Read the model definition and answer for the solid it produces. Units are mm, in the model's axes. Face numbers are marked on the shaded views. A direction names the side the tool comes from. Coordinates: 2 decimals unless noted, no trailing zeros. Loops run counter-clockwise (first coordinate to the right, second up) from the corner with the lowest first, then second, coordinate; pieces in that order, holes last.
Q1. Straight lines are drawn through the part: line 1 (Z direction, x = 103.85, y = 11.5); line 2 (X direction, y = 15, z = 31); line 3 (Y direction, x = -60.5, z = -36). For each, find the intervals that lie inside material, in ascending order.
Q2. Flat-ended cylindrical pins translate along their axes: P1, Ø4, axis at y = 11.52, z = 30.58, coming from the -X side; P2, Ø4, axis at y = 11.52, z = 30.58, coming from the +X side; P3, Ø6, axis at x = -62.5, z = -14.5, coming from the +Y side. Find the tip coordinate at first contact, or state that the pin passes through.
Q3. Section B-B (x = -41) is taken. Give the vertices of the cut face in (y, z), then the cut area to 3 significant figures.
Q4. Section A-A (z = 11) is taken. Give the vertices of the cut face in (x, y), then the cut area to 3 significant figures.
Q5. Which of the six approach directions +Z, -Z, +X, -X, +Y, -Y give full straight-line access (tool end or side, diameter ignored) to the marked faces 1 and 2?
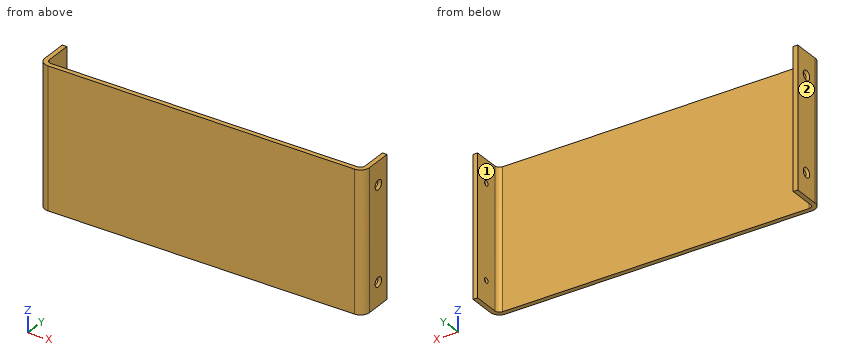
from build123d import *

# Parameters (mm, degrees)
SKETCH_1_W                            = 200
SKETCH_1_H                            = 91.16
SM_BASE_FLANGE_1_DEPTH                = 3
SM_EDGE_FLANGE_1_DEPTH                = 91.16
SM_EDGE_FLANGE_1_BEND_DEPTH           = 91.16
HOLE_WIZARD_M31_D                     = 3.4
HOLE_WIZARD_M31_DEPTH                 = 8.5
HOLE_WIZARD_M31_CSINK_D               = 6.3
HOLE_WIZARD_M31_CSINK_ANGLE           = 90
HOLE_WIZARD_M31_TIP                   = 1.021463052
HOLE_WIZARD_M31_ON_FACE_2_D           = 3.4
HOLE_WIZARD_M31_ON_FACE_2_DEPTH       = 8.5
HOLE_WIZARD_M31_ON_FACE_2_CSINK_D     = 6.3
HOLE_WIZARD_M31_ON_FACE_2_CSINK_ANGLE = 90
HOLE_WIZARD_M31_ON_FACE_2_TIP         = 1.021463052


# Sheet-metal steps are written as plain solids
with BuildPart() as part:
    # Sketch 1 → Базовая кромка1 (new body)
    with BuildSketch(Plane(origin=(0, 0, 0), x_dir=(1, 0, 0), z_dir=(0, 1, 0))):
        Rectangle(SKETCH_1_W, SKETCH_1_H)
    extrude(amount=-SM_BASE_FLANGE_1_DEPTH)

    # Ребро-кромка1 section (across the edge) → Ребро-кромка1 (add)
    with BuildSketch(Plane(origin=(-103, 0, -45.58), x_dir=(1, 0, 0), z_dir=(0, 0, 1))):
        with BuildLine():
            Line((-3, 3), (-3, 20))
            Line((-3, 20), (0, 20))
            Line((0, 20), (0, 3))
            ThreePointArc((0, 3), (0.878679656, 0.878679656), (3, 0))
            Line((3, 0), (3, -3))
            ThreePointArc((3, -3), (-1.242640687, -1.242640687), (-3, 3))
        make_face()
    extrude(amount=SM_EDGE_FLANGE_1_DEPTH)

    # Ребро-кромка1 section 2 (across the edge) → Ребро-кромка1 bend (add)
    with BuildSketch(Plane(origin=(103, 0, 45.58), x_dir=(-1, 0, 0), z_dir=(0, 0, -1))):
        with BuildLine():
            Line((-3, 3), (-3, 20))
            Line((-3, 20), (0, 20))
            Line((0, 20), (0, 3))
            ThreePointArc((0, 3), (0.878679656, 0.878679656), (3, 0))
            Line((3, 0), (3, -3))
            ThreePointArc((3, -3), (-1.242640687, -1.242640687), (-3, 3))
        make_face()
    extrude(amount=SM_EDGE_FLANGE_1_BEND_DEPTH)

    # Зенковка для  винта с плоской головкой M31
    with Locations(Plane(origin=(106, 11.522322038, 30.580016609), x_dir=(0, 1, 0), z_dir=(1, 0, 0))):
        with Locations((0, 0), (-0.022322038, -61.160016609)):
            CounterSinkHole(HOLE_WIZARD_M31_D / 2, HOLE_WIZARD_M31_CSINK_D / 2, depth=HOLE_WIZARD_M31_DEPTH, counter_sink_angle=HOLE_WIZARD_M31_CSINK_ANGLE)
            with Locations((0, 0, -(HOLE_WIZARD_M31_DEPTH + HOLE_WIZARD_M31_TIP / 2))):  # 118° drill point
                Cone(0, HOLE_WIZARD_M31_D / 2, HOLE_WIZARD_M31_TIP, mode=Mode.SUBTRACT)

    # Зенковка для  винта с плоской головкой M31 on face 2
    with Locations(Plane(origin=(-106, 11.5, -30.58), x_dir=(0, 0, -1), z_dir=(-1, 0, 0))):
        with Locations((0, 0), (-61.160016609, -0.022322038)):
            CounterSinkHole(HOLE_WIZARD_M31_ON_FACE_2_D / 2, HOLE_WIZARD_M31_ON_FACE_2_CSINK_D / 2, depth=HOLE_WIZARD_M31_ON_FACE_2_DEPTH, counter_sink_angle=HOLE_WIZARD_M31_ON_FACE_2_CSINK_ANGLE)
            with Locations((0, 0, -(HOLE_WIZARD_M31_ON_FACE_2_DEPTH + HOLE_WIZARD_M31_ON_FACE_2_TIP / 2))):  # 118° drill point
                Cone(0, HOLE_WIZARD_M31_ON_FACE_2_D / 2, HOLE_WIZARD_M31_ON_FACE_2_TIP, mode=Mode.SUBTRACT)


solid = part.part
Numbers:
1. line 1: z = -45.58 to -32.28, -28.88 to 28.88, 32.28 to 45.58
1. line 2: x = -106 to -103, 103 to 106
1. line 3: y = -3 to 0
2. P1: stops at x = -104.85
2. P2: stops at x = 104.85
2. P3: stops at y = 0
3. outline: (-3, -45.58) - (0, -45.58) - (0, 45.58) - (-3, 45.58) - close
3. area: 273 mm2
4. outline: (-106, 3) arc R6 ccw to (-100, -3) - (100, -3) arc R6 ccw to (106, 3) - (106, 20) - (103, 20) - (103, 3) arc R3 cw to (100, 0) - (-100, 0) arc R3 cw to (-103, 3) - (-103, 20) - (-106, 20) - close
4. area: 744 mm2
5. face 1: +Z, -Z, +Y
5. face 2: +Z, -Z, -X, +Y, -Y
